Source: CAD feature listing. Evaluate the final solid. Frame: model axes, mm. Coordinates: 2 decimals unless noted, no trailing zeros. Order: outer loops, then holes, each group sorted by start corner. A loop starts at its lowest first (then second) coordinate and runs counter-clockwise, first axis right, second up.
Item 1: Section B-B on z = 344. Return the cut outline in (x, y).
Item 2: Contact query for flat-ended pins moving along their axis: P1, Ø10, axis at y = 7, z = 346, coming from the +X side; P2, Ø2.5, axis at y = 0, z = 460, coming from the -X side; P3, Ø1.5, axis at y = 3.5, z = 138.5, coming from the -X side; P4, Ø1, axis at x = -6.5, z = 373.5, coming from the +Y side. Output: stop coordinate, or through.
Item 3: Ray query, line 1 (Z direction, x = 8.1, y = 0); line 2 (Y direction, x = 0.75, z = 32.5); line 3 (X direction, y = 0, z = 297.5). Return the intervals inside material, ascending.
Item 4: Section A-A on x = 0. Return the cut outline in (y, z).
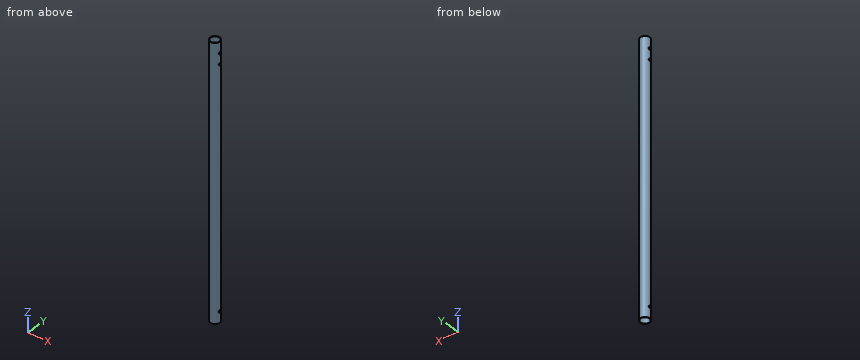
Autodesk Inventor part; units mm, degrees
ref_plane "Work Plane2" through (5.5, 0, -32) normal (1, 0, 0) x (0, 0, 1)
ref_plane "YZ Plane" through (0, 0, 0) normal (1, 0, 0) x (0, 1, 0)
ref_plane "XZ Plane" through (0, 0, 0) normal (0, 1, 0) x (-1, 0, 0)
sketch "Sketch1" plane through (0, 0, 0) normal (0, 0, 1) x (1, 0, 0)
  circle A0 centre (0, 0) radius 8
  circle A1 centre (0, 0) radius 9
  dimension "d0" = 16
  dimension "d1" = 18
extrude "Extrusion1" add sketch "Sketch1" along normal blind 500
ref_plane "Work Plane2" through (5.5, 0, -32) normal (1, 0, 0) x (0, 0, 1)
sketch "Sketch2" plane through (5.5, 0, -32) normal (1, 0, 0) x (0, 0, 1)
  circle A0 centre (52, 0) radius 2.25
  line L0 (32, -9) -> (32, 9)
  circle A1 centre (512, 0) radius 2.25
  circle A2 centre (492, 0) radius 2.25
  line L1 (532, -9) -> (532, 9)
  point P0 (32, 0)
  dimension "d4" = 4.5
  dimension "d5" = 20
  dimension "d8" = 4.5
  dimension "d9" = 4.5
  dimension "d10" = 20
  dimension "d11" = 20
extrude "Extrusion2" cut sketch "Sketch2" along normal through all both and the other way through all
properties part number "BodyTube" material "Aluminum 6061"
Answer list:
1. outline: circle Ø18 at (0, 0); hole circle Ø16 at (0, 0)
2. P1: stops at x = 8.77
2. P2: passes through
2. P3: stops at x = -8.57
2. P4: stops at y = 6.71
3. line 1: z = 0 to 17.75, 22.25 to 457.75, 462.25 to 477.75, 482.25 to 500
3. line 2: y = -8.97 to -7.96, 7.96 to 8.97
3. line 3: x = -9 to -8, 8 to 9
4. outline: (-9, 0) - (-8, 0) - (-8, 500) - (-9, 500) - close; (8, 0) - (9, 0) - (9, 500) - (8, 500) - close
